Verification items for the finished model (mm, model axes). Round coordinates to 2 decimals unless told otherwise and drop trailing zeros. Loops run counter-clockwise (first coordinate to the right, second up) from the corner with the lowest first, then second, coordinate; pieces in that order, holes last. Notation, with made-up numbers: (-38, 64) -> (-24, 64) arc R18 cw to (-24, 92) -> close; hole circle Ø7 at (86, 50). An arc over 180 degrees is marked (long way). Use CSV: the item, a comma, the result in double quotes. Start each with the question number.
Autodesk Inventor part; units mm, degrees
ref_plane "YZ Plane" through (0, 0, 0) normal (1, 0, 0) x (0, 1, 0)
ref_plane "XZ Plane" through (0, 0, 0) normal (0, 1, 0) x (-1, 0, 0)
ref_plane "XY Plane" through (0, 0, 0) normal (0, 0, 1) x (1, 0, 0)
sketch "Sketch1" plane through (0, 0, 0) normal (0, 1, 0) x (-1, 0, 0)
  line L0 (0, 0) -> (6, 0)
  line L1 (6, 0) -> (6, -6)
  line L2 (6, -6) -> (0, -6)
  line L3 (0, -6) -> (0, 0)
  line L4 (0, -6) -> (-55, -6)
  line L5 (-55, -6) -> (-55, 58)
  line L6 (-55, 58) -> (0, 58)
  line L7 (0, 58) -> (0, -6)
  dimension "d0" = 6
  dimension "d1" = 6
  dimension "d2" = 55
  dimension "d3" = 64
extrude "Extrusion1" add sketch "Sketch1" along normal blind 6
mirror "Mirror1" about plane through (55, 0, 58) normal (1, 0, 0) of "Extrusion1"
sketch "Sketch2" plane through (0, 6, 0) normal (0, 1, 0) x (1, 0, 0)
  line L0 (0, -58) -> (110, -58)
  line L1 (0, -58) -> (110, -58)
  line L2 (0, -58) -> (110, -58)
  line L3 (0, -58) -> (110, -58)
  line L4 (-6, 6) -> (-6, 0)
  line L5 (-6, 0) -> (0, 0)
  line L6 (0, 0) -> (0, -58)
  line L7 (0, -58) -> (110, -58)
  line L8 (110, 0) -> (110, -58)
  line L9 (116, 0) -> (110, 0)
  line L10 (116, 6) -> (116, 0)
  line L11 (-6, 6) -> (116, 6)
  line L12 (-6, 6) -> (116, 6)
  line L13 (-6, 6) -> (-6, 0)
  line L14 (-6, 6) -> (116, 6)
  line L15 (116, 6) -> (116, 0)
  line L16 (116, 0) -> (110, 0)
  line L17 (110, 0) -> (110, -58)
  line L18 (0, -58) -> (110, -58)
  line L19 (0, 0) -> (0, -58)
  line L20 (-6, 0) -> (0, 0)
  line L21 (-6, 6) -> (116, 6)
  line L22 (-6, 6) -> (116, 6)
  line L23 (-6, 6) -> (116, 6)
  line L24 (0, 0) -> (0, -58)
  line L25 (0, 0) -> (0, -58)
  line L26 (0, 0) -> (0, -58)
  line L27 (0, 0) -> (0, -58)
  line L28 (-6, 6) -> (-6, 0)
  line L29 (-6, 6) -> (-6, 0)
  line L30 (-6, 6) -> (-6, 0)
  line L31 (-6, 6) -> (-6, 0)
  line L32 (-6, 0) -> (0, 0)
  line L33 (-6, 0) -> (0, 0)
  line L34 (-6, 0) -> (0, 0)
  line L35 (-6, 0) -> (0, 0)
  line L36 (110, 0) -> (110, -58)
  line L37 (110, 0) -> (110, -58)
  line L38 (110, 0) -> (110, -58)
  line L39 (110, 0) -> (110, -58)
  line L40 (116, 0) -> (110, 0)
  line L41 (116, 0) -> (110, 0)
  line L42 (116, 0) -> (110, 0)
  line L43 (116, 0) -> (110, 0)
  line L44 (116, 6) -> (116, 0)
  line L45 (116, 6) -> (116, 0)
  line L46 (116, 6) -> (116, 0)
  line L47 (116, 6) -> (116, 0)
  line L48 (95, -39) -> (110, -39)
  line L49 (125, -39) -> (125, -19)
  line L50 (125, -19) -> (110, -19)
  line L51 (95, -19) -> (95, -39)
  line L52 (95, -39) -> (125, -19) construction
  line L53 (125, -39) -> (95, -19) construction
  line L54 (110, -19) -> (95, -19)
  line L55 (110, -39) -> (125, -39)
  line L56 (110, -19) -> (110, -39)
  point P0 (110, -29)
  dimension "d6" = 30
  dimension "d7" = 20
extrude "Extrusion2" cut sketch "Sketch2" against normal blind 10 contours L48 L51 L54 L8
properties part number "wall 1 for sorting"
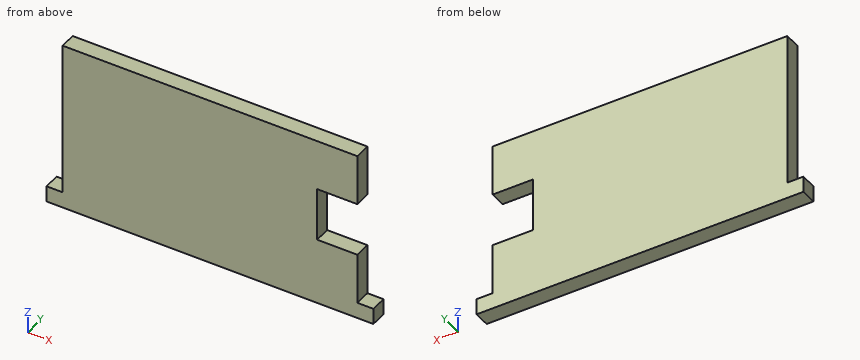
Q1. Cross-section at A-A (x = 102.5). Record the boundary of the cut face in (y, z), and give its area (3 significant figures).
Q2. Cross-section at C-C (z = 26.5). Record the boundary of the cut face in (x, y).
Q3. Depth check by flat-ended pin: pin 1 Ø2 at (y, z) = (2.5, 33.5) entering from -X; pin 2 Ø1.8 at (y, z) = (2.5, 6.5) entering from +X; pin 3 Ø1.8 at (x, y) = (-4, 1.5) entering from +Z; pin 4 Ø4 at (x, z) = (9, 18.5) entering from -Y. Enter the tip coordinate at first touch or a pass-through.
Q4. Cross-section at D-D (z = 6.5). Record the boundary of the cut face in (x, y).
Q5. Cross-section at B-B (y = 3.8). Record the boundary of the cut face in (x, z).
Q6. Thickness scan on L1, parallel to X at y = 3.15, z = 1.5; L2, parallel to X at y = 2.15, z = 22.5. Record the ranges inside material, lowest first. Write a range as from..to.
Answer list:
1,outline,"(0, -6) -> (6, -6) -> (6, 19) -> (0, 19) -> close; (0, 39) -> (6, 39) -> (6, 58) -> (0, 58) -> close"
1,area,"264 mm2"
2,outline,"(0, 0) -> (95, 0) -> (95, 6) -> (0, 6) -> close"
3,pin 1,"stops at x = 0"
3,pin 2,"stops at x = 110"
3,pin 3,"stops at z = 0"
3,pin 4,"stops at y = 0"
4,outline,"(0, 0) -> (110, 0) -> (110, 6) -> (0, 6) -> close"
5,outline,"(-6, -6) -> (116, -6) -> (116, 0) -> (110, 0) -> (110, 19) -> (95, 19) -> (95, 39) -> (110, 39) -> (110, 58) -> (0, 58) -> (0, 0) -> (-6, 0) -> close"
6,L1,"x = 0..110"
6,L2,"x = 0..95"
